Read the model definition and answer for the solid it produces. Units are mm, in the model's axes. Coordinates: 2 decimals unless noted, no trailing zeros.
from build123d import *

# Parameters (mm, degrees)
SKETCH_1_W                 = 250
SKETCH_1_H                 = 56
EXTRUDE_1_DEPTH            = 3
HOLE_WIZARD_M32_AT_2_COUNT = 2
HOLE_WIZARD_M32_AT_2_PITCH = 26
HOLE_WIZARD_M32_AT_3_COUNT = 2
HOLE_WIZARD_M32_AT_3_PITCH = 39.698866483
HOLE_WIZARD_M32_AT_4_COUNT = 2
HOLE_WIZARD_M32_AT_4_PITCH = 30
HOLE_WIZARD_M31_AT_2_COUNT = 2
HOLE_WIZARD_M31_AT_2_PITCH = 36
HOLE_WIZARD_M31_AT_3_COUNT = 2
HOLE_WIZARD_M31_AT_3_PITCH = 240
HOLE_WIZARD_M31_AT_4_COUNT = 2
HOLE_WIZARD_M31_AT_4_PITCH = 242.684980994
HOLE_WIZARD_M31_AT_5_COUNT = 2
HOLE_WIZARD_M31_AT_5_PITCH = 93
HOLE_WIZARD_M31_AT_6_COUNT = 2
HOLE_WIZARD_M31_AT_6_PITCH = 99.724620832
CUT_EXTRUDE_3_DEPTH        = 129.132743668
M3X0_51_D                  = 2.5


with BuildPart() as part:
    # Эскиз1 → Бобышка-Вытянуть1 (new body)
    with BuildSketch(Plane.XY):
        Rectangle(SKETCH_1_W, SKETCH_1_H)
    extrude(amount=EXTRUDE_1_DEPTH)

    # Эскиз8 → Зенковка для  винта с потайной головкой с внутренним шестигранником M32 (revolve, cut)
    with BuildSketch(Plane(origin=(-99, 13, 3), x_dir=(0, -1, 0), z_dir=(1, 0, 0))):
        Polygon((0, 0), (0, 3), (1.7, 3), (1.7, 1.66), (3.36, 0), align=None)
    hole_wizard_m32 = revolve(axis=Axis((-99, 13, 9.35), (0, 0, -1)), mode=Mode.SUBTRACT)

    # Зенковка для  винта с потайной головкой с внутренним шестигранником M32 at 2: Зенковка для  винта с потайной головкой с внутренним шестигранником M32 ×2
    with Locations(*[(0, -i * HOLE_WIZARD_M32_AT_2_PITCH, 0) for i in range(1, HOLE_WIZARD_M32_AT_2_COUNT)]):
        add(hole_wizard_m32, mode=Mode.SUBTRACT)

    # Зенковка для  винта с потайной головкой с внутренним шестигранником M32 at 3: Зенковка для  винта с потайной головкой с внутренним шестигранником M32 ×2
    with Locations(*[Vector(0.7556890827898176, -0.6549305384178419, 0) * (i * HOLE_WIZARD_M32_AT_3_PITCH) for i in range(1, HOLE_WIZARD_M32_AT_3_COUNT)]):
        add(hole_wizard_m32, mode=Mode.SUBTRACT)

    # Зенковка для  винта с потайной головкой с внутренним шестигранником M32 at 4: Зенковка для  винта с потайной головкой с внутренним шестигранником M32 ×2
    with Locations(*[(i * HOLE_WIZARD_M32_AT_4_PITCH, 0, 0) for i in range(1, HOLE_WIZARD_M32_AT_4_COUNT)]):
        add(hole_wizard_m32, mode=Mode.SUBTRACT)

    # Эскиз5 → Зенковка для  винта с потайной головкой с внутренним шестигранником M31 (revolve, cut)
    with BuildSketch(Plane(origin=(-120, 18, 0), x_dir=(0, 1, 0), z_dir=(1, 0, 0))):
        Polygon((0, 0), (0, 3), (1.7, 3), (1.7, 1.66), (3.36, 0), align=None)
    hole_wizard_m31 = revolve(axis=Axis((-120, 18, -6.35), (0, 0, 1)), mode=Mode.SUBTRACT)

    # Зенковка для  винта с потайной головкой с внутренним шестигранником M31 at 2: Зенковка для  винта с потайной головкой с внутренним шестигранником M31 ×2
    with Locations(*[(0, -i * HOLE_WIZARD_M31_AT_2_PITCH, 0) for i in range(1, HOLE_WIZARD_M31_AT_2_COUNT)]):
        add(hole_wizard_m31, mode=Mode.SUBTRACT)

    # Зенковка для  винта с потайной головкой с внутренним шестигранником M31 at 3: Зенковка для  винта с потайной головкой с внутренним шестигранником M31 ×2
    with Locations(*[(i * HOLE_WIZARD_M31_AT_3_PITCH, 0, 0) for i in range(1, HOLE_WIZARD_M31_AT_3_COUNT)]):
        add(hole_wizard_m31, mode=Mode.SUBTRACT)

    # Зенковка для  винта с потайной головкой с внутренним шестигранником M31 at 4: Зенковка для  винта с потайной головкой с внутренним шестигранником M31 ×2
    with Locations(*[Vector(0.9889363528682976, -0.14834045293024464, 0) * (i * HOLE_WIZARD_M31_AT_4_PITCH) for i in range(1, HOLE_WIZARD_M31_AT_4_COUNT)]):
        add(hole_wizard_m31, mode=Mode.SUBTRACT)

    # Зенковка для  винта с потайной головкой с внутренним шестигранником M31 at 5: Зенковка для  винта с потайной головкой с внутренним шестигранником M31 ×2
    with Locations(*[(i * HOLE_WIZARD_M31_AT_5_PITCH, 0, 0) for i in range(1, HOLE_WIZARD_M31_AT_5_COUNT)]):
        add(hole_wizard_m31, mode=Mode.SUBTRACT)

    # Зенковка для  винта с потайной головкой с внутренним шестигранником M31 at 6: Зенковка для  винта с потайной головкой с внутренним шестигранником M31 ×2
    with Locations(*[Vector(0.9325680982740896, -0.36099410255771214, 0) * (i * HOLE_WIZARD_M31_AT_6_PITCH) for i in range(1, HOLE_WIZARD_M31_AT_6_COUNT)]):
        add(hole_wizard_m31, mode=Mode.SUBTRACT)

    # Эскиз7 → Вырез-Вытянуть3 (cut, through all)
    with BuildSketch(Plane.XY.offset(3)):
        with BuildLine():
            Line((6.030531049, 21.7), (24.030531049, 21.7))
            ThreePointArc((24.030531049, 21.7), (25.730531049, 20), (24.030531049, 18.3))
            Line((24.030531049, 18.3), (6.030531049, 18.3))
            ThreePointArc((6.030531049, 18.3), (4.330531049, 20), (6.030531049, 21.7))
        make_face()
        with BuildLine():
            Line((46.030531049, 21.7), (64.030531049, 21.7))
            ThreePointArc((64.030531049, 21.7), (65.730531049, 20), (64.030531049, 18.3))
            Line((64.030531049, 18.3), (46.030531049, 18.3))
            ThreePointArc((46.030531049, 18.3), (44.330531049, 20), (46.030531049, 21.7))
        make_face()
        with BuildLine():
            Line((86.030531049, 21.7), (104.030531049, 21.7))
            ThreePointArc((104.030531049, 21.7), (105.730531049, 20), (104.030531049, 18.3))
            Line((104.030531049, 18.3), (86.030531049, 18.3))
            ThreePointArc((86.030531049, 18.3), (84.330531049, 20), (86.030531049, 21.7))
        make_face()
        with BuildLine():
            Line((6.030531049, -18.3), (24.030531049, -18.3))
            ThreePointArc((24.030531049, -18.3), (25.730531049, -20), (24.030531049, -21.7))
            Line((24.030531049, -21.7), (6.030531049, -21.7))
            ThreePointArc((6.030531049, -21.7), (4.330531049, -20), (6.030531049, -18.3))
        make_face()
        with BuildLine():
            Line((46.030531049, -18.3), (64.030531049, -18.3))
            ThreePointArc((64.030531049, -18.3), (65.730531049, -20), (64.030531049, -21.7))
            Line((64.030531049, -21.7), (46.030531049, -21.7))
            ThreePointArc((46.030531049, -21.7), (44.330531049, -20), (46.030531049, -18.3))
        make_face()
        with BuildLine():
            Line((86.030531049, -18.3), (104.030531049, -18.3))
            ThreePointArc((104.030531049, -18.3), (105.730531049, -20), (104.030531049, -21.7))
            Line((104.030531049, -21.7), (86.030531049, -21.7))
            ThreePointArc((86.030531049, -21.7), (84.330531049, -20), (86.030531049, -18.3))
        make_face()
    extrude(amount=-CUT_EXTRUDE_3_DEPTH, mode=Mode.SUBTRACT)

    # Отверстие обработанное метчиком M3x0.51 (through all)
    with Locations(Plane.XY.offset(3)):
        with Locations((-108, 18.5), (-108, -18.5), (-39, -18.5), (-39, 18.5)):
            Hole(M3X0_51_D / 2)


solid = part.part
Q1. The part is cut by section A-A, the plane z = 2.3. State how many separate pieces and enclosed holes the cut face has, then the cut area to 3 significant figures.
Q2. Straight lines are drawn through the part: L1, parallel to X at y = 13, z = 0.85; L2, parallel to Y at x = -108, z = 2; L3, parallel to Y at x = 101.5, z = 2.35. For each, find the intervals that lie inside material, in ascending order.
Q3. This flat-tipped pin is pushed along its axis until it touches: P1, Ø4.5, axis at x = -99, y = -13, coming from the +Z side. Where does it stop, or does it pass through?
Computed values:
1. separate pieces: 1
1. enclosed holes: 20
1. area: 13,400 mm2
2. L1: x = -125 to -100.7, -97.3 to -70.7, -67.3 to 125
2. L2: y = -28 to -19.75, -17.25 to 17.25, 19.75 to 28
2. L3: y = -28 to -21.7, -18.3 to 18.3, 21.7 to 28
3. P1: stops at z = 1.89
